The model under review builds one solid part; all positions refer to its coordinate system, in mm. A direction names the side the tool comes from. Coordinates: 2 decimals unless noted, no trailing zeros. Loops run counter-clockwise (first coordinate to the right, second up) from the corner with the lowest first, then second, coordinate; pieces in that order, holes last. Notation, with made-up numbers: (41, 60) - (84, 60) arc R14 cw to (84, 69) - close; hole circle Ø1 at (54.5, -40). An arc over 180 degrees is marked (long way). Answer in a Markdown table with one row per item. Add a question column.
(1) For line 1 along Z through (x, y) = (7.75, 3.75); line 2 along Y through (x, z) = (0.25, -10.75) (3 decimals); line 3 along X through (y, z) = (-0.75, -0.75), list the stretches that pass through material, from the lowest coordinate up.
(2) We need section A-A on x = 0. Write out the cut boundary in (y, z) (3 decimals).
(3) Mouldability with a two-part tool opening along Y and no side actions: class faces 1 (the flat face through (11, -2, -11)), 2 (the flat face through (4, -4, -10)), 3 (the flat face through (3.125, 1.838, -4.888)) as +Y half, -Y half, draft (parallel to the pull), parting line (faces both ways), or undercut.
(4) We need section C-C on y = -3.25. Write out the cut boundary in (x, z).
(5) For P1, Ø4.5, axis at x = -0.5, z = -8, coming from the -Y side; P2, Ø6, axis at x = -4.5, z = -9, coming from the +Y side; P3, Ø1.3, axis at x = 0.5, z = -2, coming from the +Y side; P4, Ø6, axis at x = -1.5, z = -5, coming from the -Y side, all flat-tipped, find the tip position at first contact; note any pin that passes through.
(6) We need section D-D on z = 0.5. Write out the cut boundary in (x, y) (3 decimals), plus the area to 3 significant figures.
(7) We need section B-B on z = -6. Write out the cut boundary in (x, y) (3 decimals), plus the area to 3 significant figures.
(8) Machinability: for faces 4 (the cylindrical face through (-1.08, -4.88, -4.93)), 5 (the flat face through (-3.125, -1.838, -4.888)), 6 (the flat face through (0, -4, 3)), 7 (the flat face through (11, 2, -11)), which of the approach directions +Z, -Z, +X, -X, +Y, -Y give a long, thin tool a straight path to every point of the face, cutting with its end or side? Answer none if there is none.
Autodesk Inventor part; units mm, degrees
ref_plane "YZ Plane" through (0, 0, 0) normal (1, 0, 0) x (0, 1, 0)
ref_plane "XZ Plane" through (0, 0, 0) normal (0, 1, 0) x (-1, 0, 0)
ref_plane "XY Plane" through (0, 0, 0) normal (0, 0, 1) x (1, 0, 0)
sketch "Sketch1" plane through (0, 0, 0) normal (0, 0, 1) x (1, 0, 0)
  circle A0 centre (0, 0) radius 9
  circle A1 centre (0, 0) radius 5
  line L0 (4.1858, 0) -> (2.0929, -3.625)
  line L1 (2.0929, -3.625) -> (-2.0929, -3.625)
  line L2 (-2.0929, -3.625) -> (-4.1858, 0)
  line L3 (-4.1858, 0) -> (-2.0929, 3.625)
  line L4 (-2.0929, 3.625) -> (2.0929, 3.625)
  line L5 (2.0929, 3.625) -> (4.1858, 0)
  dimension "d1" = 18
  dimension "d2" = 10
  dimension "d3" = 7.25
extrude "Extrusion2" add sketch "Sketch1" against normal blind 10 contours A1
extrude "Extrusion4" add sketch "Sketch1" along normal blind 3 contours A0 | A1
sketch "Sketch6" plane through (0, 0, -10) normal (0, 0, -1) x (-1, 0, 0)
  circle A0 centre (0, 0) radius 9
  circle A1 centre (0, 0) radius 5
  line L0 (0, 0) -> (-9, 0) construction
  arc A2 (-8.775, 2) -> (-8.775, -2) centre (0, 0) ccw
  line L1 (-8.775, -2) -> (-12.275, -2)
  line L2 (-12.275, -2) -> (-12.275, 2)
  line L3 (-12.275, 2) -> (-8.775, 2)
  line L4 (-4.1858, 0) -> (-2.0929, 3.625)
  line L5 (-2.0929, 3.625) -> (2.0929, 3.625)
  line L6 (2.0929, 3.625) -> (4.1858, 0)
  line L7 (4.1858, 0) -> (2.0929, -3.625)
  line L8 (2.0929, -3.625) -> (-2.0929, -3.625)
  line L9 (-2.0929, -3.625) -> (-4.1858, 0)
  circle A3 centre (0, 0) radius 5
  dimension "d20" = 3.5
  dimension "d21" = 4
extrude "Extrusion7" add sketch "Sketch6" along normal blind 3 contours A0 | A0 L1 L2 L3 | A1
properties part number "movingSpindle"
Outcome:
| question | item | result |
|---|---|---|
| 1 | line 1 | -13 to -10, 0 to 3 |
| 1 | line 2 | -8.997 to -3.625, 3.625 to 8.997 |
| 1 | line 3 | -4.94 to -3.75, 3.75 to 4.94 |
| 2 | outline | (-9, -13) - (-3.625, -13) - (-3.625, 3) - (-9, 3) - (-9, 0) - (-5, 0) - (-5, -10) - (-9, -10) - close; (3.625, -13) - (9, -13) - (9, -10) - (5, -10) - (5, 0) - (9, 0) - (9, 3) - (3.625, 3) - close |
| 3 | face 1 | -Y half |
| 3 | face 2 | draft |
| 3 | face 3 | undercut |
| 4 | outline | (-8.39, -13) - (-2.31, -13) - (-2.31, 3) - (-8.39, 3) - (-8.39, 0) - (-3.8, 0) - (-3.8, -10) - (-8.39, -10) - close; (2.31, -13) - (8.39, -13) - (8.39, -10) - (3.8, -10) - (3.8, 0) - (8.39, 0) - (8.39, 3) - (2.31, 3) - close |
| 5 | P1 | y = -9 |
| 5 | P2 | y = 8.84 |
| 5 | P3 | y = 5 |
| 5 | P4 | y = -5 |
| 6 | outline | circle Ø18 at (0, 0); hole (-4.186, 0) - (-2.093, -3.625) - (2.093, -3.625) - (4.186, 0) - (2.093, 3.625) - (-2.093, 3.625) - close |
| 6 | area | 209 mm² |
| 7 | outline | circle Ø10 at (0, 0); hole (-4.186, 0) - (-2.093, -3.625) - (2.093, -3.625) - (4.186, 0) - (2.093, 3.625) - (-2.093, 3.625) - close |
| 7 | area | 33.0 mm² |
| 8 | face 4 | none |
| 8 | face 5 | +Z, -Z |
| 8 | face 6 | +Z, +X, -X, +Y, -Y |
| 8 | face 7 | +Z, -Z, +X, +Y |
